from build123d import *

# Parameters (mm, degrees)
F0_W      = 444.5
F0_H      = 203.2
F1_DEPTH  = 12.7
F2_W      = 114.3
F2_H      = 177.8
F3_DEPTH  = 12.7
F5_D      = 9.525
F6_W      = 203.2
F6_H      = 9.652
F6_W_2    = 6.35
F6_H_2    = 63.5
F6_W_3    = 196.85
F7_DEPTH  = 511.048
F9_DEPTH  = 106.427
F10_W     = 228.6
F10_H     = 203.2
F11_DEPTH = 19.05
F13_D     = 14.2875
F13_DEPTH = 31.75
F13_TIP   = 4.2923980472


# Not quite as in the source:
# - a length typed as a fraction of an inch, garbled in the dataset ("3 / 203.2 mm" for 3/8 in), is restored


with BuildPart() as f1:
    # F0 (on Top) → F1 (new body)
    with BuildSketch(Plane.XY):
        Rectangle(F0_W, F0_H)
    extrude(amount=F1_DEPTH)

    # F2 (on face) → F3 (join)
    with BuildSketch(Plane.XY.offset(12.7)):
        with Locations((-152.4, 0)):
            Rectangle(F2_W, F2_H)
    extrude(amount=F3_DEPTH)

    # F5 (through all)
    with Locations(Plane.XY.offset(25.4)):
        with Locations((-190.5, 61.976), (-114.3, 61.976), (-114.3, -61.976), (-190.5, -61.976)):
            Hole(F5_D / 2)

    # F6 (on face) → F7 (join)
    with BuildSketch(Plane(origin=(0, 0, 0), x_dir=(1, 0, 0), z_dir=(0, 0, -1))):
        with Locations((-101.6, 0)):
            Rectangle(F6_W, F6_H)
        with Locations((3.175, 0)):
            Rectangle(F6_W_2, F6_H)
        with Locations((3.175, -36.576)):
            Rectangle(F6_W_2, F6_H_2)
        with Locations((104.775, 0)):
            Rectangle(F6_W_3, F6_H)
        with Locations((3.175, 36.576)):
            Rectangle(F6_W_2, F6_H_2)
    extrude(amount=F7_DEPTH)

    # F8 (on face) → F9 (cut, through all)
    with BuildSketch(Plane.XZ.offset(4.826)):
        Polygon((203.2, -88.9), (25.4, -511.048), (203.2, -511.048), align=None)
    extrude(amount=-F9_DEPTH, mode=Mode.SUBTRACT)

    # F10 (on face) → F11 (join)
    with BuildSketch(Plane(origin=(0, 0, -511.048), x_dir=(1, 0, 0), z_dir=(0, 0, -1))):
        with Locations((-88.9, 0)):
            Rectangle(F10_W, F10_H)
    extrude(amount=F11_DEPTH)

    # F13
    with Locations(Plane(origin=(0, 0, -530.098), x_dir=(1, 0, 0), z_dir=(0, 0, -1))):
        with Locations((-184.15, 82.55), (-95.25, 82.55), (-95.25, -82.55), (-184.15, -82.55)):
            Hole(F13_D / 2, depth=F13_DEPTH)
            with Locations((0, 0, -(F13_DEPTH + F13_TIP / 2))):  # 118° drill point
                Cone(0, F13_D / 2, F13_TIP, mode=Mode.SUBTRACT)


solid = f1.part
The listing builds one solid part. Answer for the finished solid, in the listing's coordinates (mm). A direction names the side the tool comes from. Coordinates: 2 decimals unless noted, no trailing zeros. Write each loop counter-clockwise with the first axis right and the second up, starting at its lowest first coordinate (ties: lowest second). Pieces come first, ordered by that corner, then holes. Notation, with made-up numbers: M -23.5,-19 L 23.5,-19 A21 ccw 23.5,20 Z; hole C 37,66 d1. An arc over 180 degrees is marked long. Use one line per item in the form item = value.
Item 1: Find the intervals of material crossed by probe 1 along X at (y, z) = (-82, -516); probe 2 along Y at (x, z) = (-114.3, 19.75); probe 3 along Z at (x, y) = (23, 68.5), in increasing order.
Model answer:
probe_1 = -203.2 to -191.27, -177.03 to -102.37, -88.13 to 25.4
probe_2 = -88.9 to -66.74, -57.21 to 57.21, 66.74 to 88.9
probe_3 = -530.1 to -511.05, 0 to 12.7
Item 2: Find section A-A, the plane y = 82.55. Give the vertices of the cut face in (x, z).
Model answer:
outline = M -222.25,0 L 222.25,0 L 222.25,12.7 L -95.25,12.7 L -95.25,25.4 L -209.55,25.4 L -209.55,12.7 L -222.25,12.7 Z; M -203.2,-530.1 L -191.29,-530.1 L -191.29,-511.05 L -203.2,-511.05 Z; M -177.01,-530.1 L -102.39,-530.1 L -102.39,-511.05 L -177.01,-511.05 Z; M -88.11,-530.1 L 25.4,-530.1 L 25.4,-511.05 L -88.11,-511.05 Z
Item 3: For faces 1 (the face through (25.4, 1, -520)), 2 (the face through (82, 4.826, -195)), 3 (the face through (-209.55, -1, 19)), 4 (the face through (-100, -4.826, -252)), 5 (the face through (84, -4.826, -195)), determine the directions among +Z, -Z, +X, -X, +Y, -Y from which every point of the face is accessible in a straight line to the end or side of a thin tool.
Model answer:
face_1 = -Z, +X, +Y, -Y
face_2 = +X, +Y
face_3 = +Z, -X, +Y, -Y
face_4 = -X, -Y
face_5 = +X, -Y
Item 4: Given P1, Ø10, axis at y = -18, z = 21, coming from the +X side; P2, Ø10, axis at x = -9, z = -283.5, coming from the -Y side; P3, Ø5, axis at y = 13, z = -106, coming from the +X side, each flat-ended and moving along its own axis, determine where each tip first touches the part or whether it passes through.
Model answer:
P1 = -95.25
P2 = -4.83
P3 = 6.35
Item 5: Find section D-D, the plane z = -234.5. Give the vertices of the cut face in (x, y).
Model answer:
outline = M -203.2,-4.83 L 0,-4.83 L 0,-68.33 L 6.35,-68.33 L 6.35,-4.83 L 141.88,-4.83 L 141.88,4.83 L 6.35,4.83 L 6.35,68.33 L 0,68.33 L 0,4.83 L -203.2,4.83 Z
Item 6: Find section B-B, the plane y = 12.5. Give the vertices of the cut face in (x, z), plus the area to 3 significant figures.
Model answer:
outline = M -222.25,0 L 0,0 L 0,-511.05 L -203.2,-511.05 L -203.2,-530.1 L 25.4,-530.1 L 25.4,-511.05 L 6.35,-511.05 L 6.35,0 L 222.25,0 L 222.25,12.7 L -95.25,12.7 L -95.25,25.4 L -209.55,25.4 L -209.55,12.7 L -222.25,12.7 Z
area = 14,700 mm2
Item 7: Find section C-C, the plane x = -29.5. Give the vertices of the cut face in (y, z).
Model answer:
outline = M -101.6,-530.1 L 101.6,-530.1 L 101.6,-511.05 L 4.83,-511.05 L 4.83,0 L 101.6,0 L 101.6,12.7 L -101.6,12.7 L -101.6,0 L -4.83,0 L -4.83,-511.05 L -101.6,-511.05 Z
Item 8: The mould has two halves that part along X. Classify faces 6 (the face through (115.545, -0.068, -297.019)), 7 (the face through (-153, 1, 25.4)), 8 (the face through (-177.013, 82.236, -520.44)): released by +X, released by -X, zero draft, split by the parting line, or undercut.
Model answer:
face_6 = released by +X
face_7 = zero draft
face_8 = undercut
